from build123d import *

# Parameters (mm, degrees)
CROQUIS1_W              = 80.8
CROQUIS1_H              = 25
CROQUIS1_R              = 1.5
SALIENTE_EXTRUIR1_DEPTH = 5
CROQUIS1_3_W            = 80.8
CROQUIS1_3_H            = 5
SALIENTE_EXTRUIR2_DEPTH = 26
CROQUIS1_4_R            = 1.5
SALIENTE_EXTRUIR3_DEPTH = 5
SALIENTE_EXTRUIR4_DEPTH = 26
CROQUIS3_R              = 2.25
CORTAR_EXTRUIR1_DEPTH   = 26
SALIENTE_EXTRUIR5_DEPTH = 21
CORTAR_EXTRUIR2_DEPTH   = 21
CROQUIS7_W              = 36.882036787
CROQUIS7_H              = 40.226112096
CORTAR_EXTRUIR3_DEPTH   = 90
CROQUIS8_W              = 35.258342774
CROQUIS8_H              = 26
SALIENTE_EXTRUIR6_DEPTH = 0.5


with BuildPart() as part:
    # Croquis1 → Saliente-Extruir1 (new body)
    with BuildSketch(Plane(origin=(0, 0, 0), x_dir=(1, 0, 0), z_dir=(0, 1, 0))):
        with Locations((0, -10)):
            Rectangle(CROQUIS1_W, CROQUIS1_H)
        with Locations((15.4, -12.5)):
            Circle(CROQUIS1_R, mode=Mode.SUBTRACT)
        with Locations((-15.4, -12.5)):
            Circle(CROQUIS1_R, mode=Mode.SUBTRACT)
    extrude(amount=SALIENTE_EXTRUIR1_DEPTH)

    # Croquis1_3 → Saliente-Extruir2 (add)
    with BuildSketch(Plane(origin=(0, 0, 0), x_dir=(1, 0, 0), z_dir=(0, 1, 0))):
        Rectangle(CROQUIS1_3_W, CROQUIS1_3_H)
    extrude(amount=SALIENTE_EXTRUIR2_DEPTH)

    # Croquis1_4 → Saliente-Extruir3 (add)
    with BuildSketch(Plane(origin=(0, 0, 0), x_dir=(1, 0, 0), z_dir=(0, 1, 0))):
        Polygon((-45.4, -2.5), (-40.4, -2.5), (-40.4, 2.5), (-40.4, 37.5), (-45.4, 37.5), align=None)
        Polygon((-40.4, -22.5), (-40.4, -2.5), (-45.4, -2.5), (-45.4, 37.5), (-66.4, 37.5), (-66.4, -22.5), align=None)
        with Locations((-55.4, 12.5)):
            Circle(CROQUIS1_4_R, mode=Mode.SUBTRACT)
        Polygon((45.4, -2.5), (40.4, -2.5), (40.4, -22.5), (66.4, -22.5), (66.4, 37.5), (45.4, 37.5), align=None)
        with Locations((55.4, 12.5)):
            Circle(CROQUIS1_4_R, mode=Mode.SUBTRACT)
        Polygon((40.4, 2.5), (40.4, -2.5), (45.4, -2.5), (45.4, 37.5), (40.4, 37.5), align=None)
    extrude(amount=SALIENTE_EXTRUIR3_DEPTH)

    # Croquis1_5 → Saliente-Extruir4 (add)
    with BuildSketch(Plane(origin=(0, 0, 0), x_dir=(1, 0, 0), z_dir=(0, 1, 0))):
        Polygon((-45.4, -2.5), (-40.4, -2.5), (-40.4, 2.5), (-40.4, 37.5), (-45.4, 37.5), align=None)
        Polygon((40.4, 2.5), (40.4, -2.5), (45.4, -2.5), (45.4, 37.5), (40.4, 37.5), align=None)
    extrude(amount=SALIENTE_EXTRUIR4_DEPTH)

    # Croquis3 → Cortar-Extruir1 (cut)
    with BuildSketch(Plane.XY.offset(2.5)):
        with Locations((-23.5, 10)):
            Circle(CROQUIS3_R)
        with Locations((24, 10)):
            Circle(CROQUIS3_R)
    extrude(amount=-CORTAR_EXTRUIR1_DEPTH, mode=Mode.SUBTRACT)

    # Croquis4 → Saliente-Extruir5 (add)
    with BuildSketch(Plane(origin=(0, 5, 0), x_dir=(1, 0, 0), z_dir=(0, 1, 0))):
        Polygon((-45.4, -0.5), (-45.4, -2.5), (-43.4, -2.5), (-64.4, -22.5), (-66.4, -22.5), (-66.4, -20.5), align=None)
    saliente_extruir5 = extrude(amount=SALIENTE_EXTRUIR5_DEPTH)

    # Croquis5 → Cortar-Extruir2 (cut)
    with BuildSketch(Plane(origin=(-19.393579073, 0, -20.363258026), x_dir=(0.724137931, 0, -0.689655172), z_dir=(0.689655172, 0, 0.724137931))):
        Polygon((-62.151724138, 5), (-33.151724138, 26), (-26.486949689, 30.82621598), (-82.759555013, 33.403814281), (-84.060607683, 5), align=None)
    cortar_extruir2 = extrude(amount=-CORTAR_EXTRUIR2_DEPTH, mode=Mode.SUBTRACT)

    # Simetr_a1: Saliente-Extruir5 across plane
    add(saliente_extruir5.mirror(Plane(origin=(0, 0, 0), x_dir=(0, 0, 1), z_dir=(1, 0, 0))))

    # Simetr_a2: Cortar-Extruir2 across plane
    add(cortar_extruir2.mirror(Plane(origin=(0, 0, 0), x_dir=(0, 0, 1), z_dir=(1, 0, 0))), mode=Mode.SUBTRACT)

    # Croquis7 → Cortar-Extruir3 (cut)
    with BuildSketch(Plane(origin=(0, 0, -37.5), x_dir=(-1, 0, 0), z_dir=(0, 0, -1))):
        with Locations((-58.841018394, 20.113056048)):
            Rectangle(CROQUIS7_W, CROQUIS7_H)
    extrude(amount=-CORTAR_EXTRUIR3_DEPTH, mode=Mode.SUBTRACT)

    # Croquis8 → Saliente-Extruir6 (add)
    with BuildSketch(Plane(origin=(-40.4, 0, 0), x_dir=(0, 0, -1), z_dir=(1, 0, 0))):
        with Locations((20, 13)):
            Rectangle(CROQUIS8_W, CROQUIS8_H)
    extrude(amount=SALIENTE_EXTRUIR6_DEPTH)


solid = part.part
The model under review builds one solid part; all positions refer to its coordinate system, in mm. A direction names the side the tool comes from. Round coordinates to 2 decimals unless told otherwise and drop trailing zeros. Loops run counter-clockwise (first coordinate to the right, second up) from the corner with the lowest first, then second, coordinate; pieces in that order, holes last. Notation, with made-up numbers: M -39,81 L -29,81 A36 ccw -29,119 Z; hole C -13,88 d10. An arc over 180 degrees is marked long. Answer as CSV lines item,"result". Start each with the question number.
Item 1: Consider section D-D (y = 23). Write out the cut boundary in (x, z).
Item 2: Insertion check: P1, Ø3.5, axis at x = -15.4, z = 12.5, coming from the +Y side; P2, Ø8, axis at x = -52.5, z = 6, coming from the +Y side; P3, Ø10, axis at y = 22, z = -26.5, coming from the +X side. Each pin has a flat end and moves straight along its axis. Give the tip position at first contact, or say it passes through.
Item 3: Mouldability with a two-part tool opening along Z and no side actions: class faces 1 (the face through (-56.6, 2.5, -11.6)), 2 (the face through (-21.354, 10.676, 0.035)), 3 (the face through (13.9, 2.46, 12.43)), 4 (the face through (-2, 15, 2.5)) as released by +Z, released by -Z, zero draft, split by the parting line, or undercut.
Item 4: Wall thickness on line 1 (Z direction, x = -55.4, y = 2.75); line 2 (Z direction, x = -15.4, y = 2.75); line 3 (Y direction, x = 24, z = 1): over which ranges is each line inside the solid? List them lowest first. Write a range as [from, to].
Item 5: Consider section A-A (z = -12.5). Write out the cut boundary in (x, y), then the cut area to 3 significant figures.
Item 6: For faces 5 (the face through (-13, 5, 12)), 6 (the face through (-47, 4, -37.5)), 7 (the face through (-51.366, 10.673, 6.182)), 8 (the face through (-39.9, 13, -20)), 9 (the face through (-14, 2, 22.5)), list the 3-axis set-ups (+Z, -Z, +X, -X, +Y, -Y) from which the entire face can be reached by the end or side of a thin tool; tool diameter is ignored.
Item 7: Consider section B-B (x = 24). Write out the cut boundary in (y, z), then the cut area to 4 significant figures.
Item 8: Consider section C-C (z = 12.5). Write out the cut boundary in (x, y).
Answer:
1,outline,"M -48.35,3.31 L -45.4,0.5 L -45.4,-37.5 L -40.4,-37.5 L -40.4,-37.63 L -39.9,-37.63 L -39.9,-2.5 L 40.4,-2.5 L 40.4,2.5 L -43.4,2.5 L -46.4,5.36 Z"
2,P1,"stops at y = 5"
2,P2,"stops at y = 22.3"
2,P3,"stops at x = -39.9"
3,face 1,"undercut"
3,face 2,"zero draft"
3,face 3,"undercut"
3,face 4,"released by +Z"
4,line 1,"z = [-37.5, -14], [-11, 22.5]"
4,line 2,"z = [-2.5, 11], [14, 22.5]"
4,line 3,"y = [0, 7.75], [12.25, 26]"
5,outline,"M -66.4,0 L -56.9,0 L -56.9,5 L -66.4,5 Z; M -53.9,0 L -39.9,0 L -39.9,26 L -45.4,26 L -45.4,5 L -53.9,5 Z"
5,area,"233 mm^2"
6,face 5,"+Z, +X, +Y"
6,face 6,"-Z, -X, +Y, -Y"
6,face 7,"-Z, -X, +Y"
6,face 8,"-Z, +X, +Y, -Y"
6,face 9,"+Z, +X, -X, +Y, -Y"
7,outline,"M 0,-2.5 L 7.75,-2.5 L 7.75,2.5 L 5,2.5 L 5,22.5 L 0,22.5 Z; M 12.25,-2.5 L 26,-2.5 L 26,2.5 L 12.25,2.5 Z"
7,area,"207.5 mm^2"
8,outline,"M -66.4,0 L -16.9,0 L -16.9,5 L -53.9,5 L -53.9,15.5 L -58,13.35 L -58,5 L -66.4,5 Z; M -13.9,0 L 13.9,0 L 13.9,5 L -13.9,5 Z; M 16.9,0 L 40.4,0 L 40.4,5 L 16.9,5 Z"
